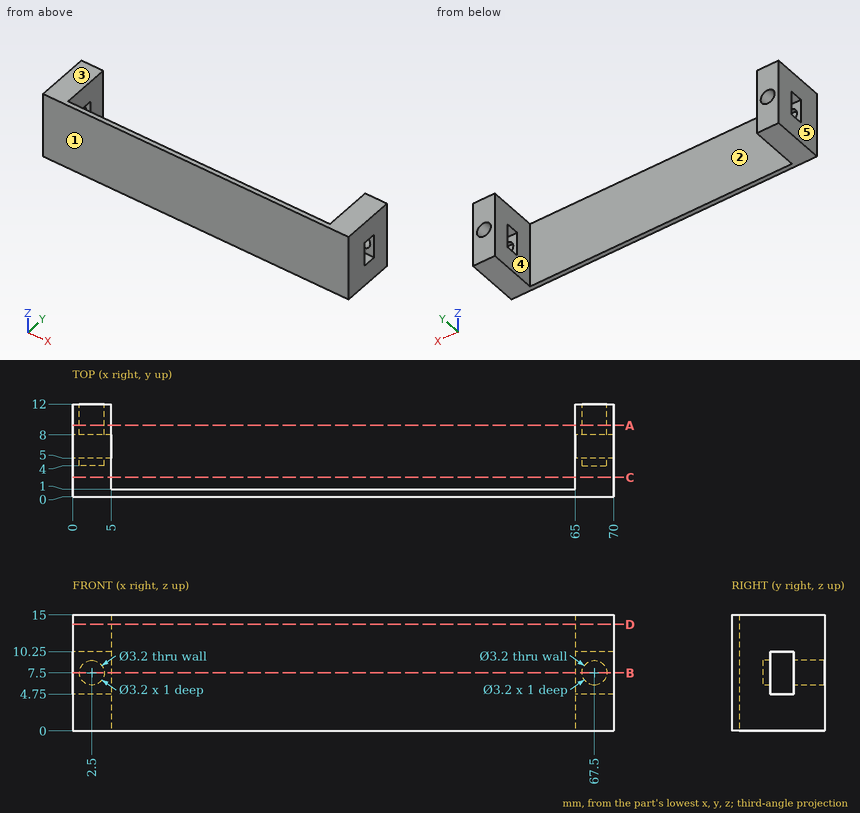
Study the drawing (mm; zero at the part's minimum x, y, z) and answer. A direction names the side the tool comes from. Coordinates: 2 decimals unless noted, no trailing zeros. Write each loop counter-clockwise with the first axis right and the second up, starting at its lowest first coordinate (ties: lowest second). Pieces come first, ordered by that corner, then holes. Notation, with made-up numbers: (48.5, 33) - (106.5, 33) arc R13 ccw to (106.5, 50) - close; hole circle Ø4 at (0.5, 89.25). An arc over 180 degrees is marked (long way). Answer as a JSON object with one key per item and string values. Group by question number.
1. A cutting plane is placed at C-C (y = 2.5). Determine the outline of the cut face in (x, z).
2. Consider L1, parallel to X at y = 10.3, z = 7.5; L2, parallel to X at y = 9.5, z = 3; L3, parallel to X at y = 10, z = 6.75. Determine where each line is inside the solid, lowest interval first. Write a range as [from, to].
3. A cutting plane is placed at A-A (y = 9.25). Determine the outline of the cut face in (x, z), plus the area to 3 significant figures.
4. Each of these flat-tipped pins is pushed along its axis until it touches: P1, Ø2.5, axis at x = 67.5, z = 7.5, coming from the +Y side; P2, Ø7.5, axis at x = 28.5, z = 11, coming from the +Y side. Where does it stop, or does it pass through?
5. The mould has two halves that part along X. Classify the marked faces 3, 4 and 5: +X half, -X half, draft (parallel to the pull), parting line (faces both ways), or undercut.
6. A cutting plane is placed at B-B (z = 7.5). Give the number of separate pieces and of enclosed holes in the cut face, plus the area to 3 significant figures.
7. A cutting plane is placed at D-D (z = 13.75). Determine the outline of the cut face in (x, y).
8. Which of the six approach directions +Z, -Z, +X, -X, +Y, -Y give full straight-line access (tool end or side, diameter ignored) to the marked faces 1 and 2?
Worked out:
{
 "1": {"outline": "(0, 0) - (5, 0) - (5, 15) - (0, 15) - close; (65, 0) - (70, 0) - (70, 15) - (65, 15) - close"},
 "2": {"L1": "x = [0, 0.9], [4.1, 5], [65, 65.9], [69.1, 70]", "L2": "x = [0, 5], [65, 70]", "L3": "x = [0, 1.09], [3.91, 5], [65, 66.09], [68.91, 70]"},
 "3": {"outline": "(0, 0) - (5, 0) - (5, 15) - (0, 15) - close; (65, 0) - (70, 0) - (70, 15) - (65, 15) - close; hole circle Ø3.2 at (2.5, 7.5); hole circle Ø3.2 at (67.5, 7.5)", "area": "134 mm²"},
 "4": {"P1": "stops at y = 4", "P2": "stops at y = 1"},
 "5": {"face 3": "draft", "face 4": "undercut", "face 5": "-X half"},
 "6": {"separate pieces": "5", "enclosed holes": "0", "area": "118 mm²"},
 "7": {"outline": "(0, 0) - (70, 0) - (70, 12) - (65, 12) - (65, 1) - (5, 1) - (5, 12) - (0, 12) - close"},
 "8": {"face 1": "+Z, -Z, +X, -X, -Y", "face 2": "+Z, -Z, +Y"}
}
